Check sheet for the modelled part. Datum: model origin and axes. Units: mm. Round coordinates to 2 decimals unless told otherwise and drop trailing zeros. Loops run counter-clockwise (first coordinate to the right, second up) from the corner with the lowest first, then second, coordinate; pieces in that order, holes last. Notation, with made-up numbers: (6, -33.75) - (22, -33.75) arc R24 cw to (22, -17.75) - close; hole circle Ø5 at (-5, 16). An arc over 180 degrees is marked (long way). Put each result on its own line as item: value.
```python
from build123d import *

# Parameters (mm, degrees)
SKETCH1_W           = 115
SKETCH1_H           = 15
BOSS_EXTRUDE1_DEPTH = 0.5
SKETCH2_W           = 115
SKETCH2_H           = 10
CUT_EXTRUDE1_DEPTH  = 0.1
SKETCH3_W           = 0.4
SKETCH3_H           = 10
CUT_EXTRUDE2_DEPTH  = 0.4
LPATTERN3_COUNT     = 150
LPATTERN3_PITCH     = 0.8
SKETCH4_W           = 115
SKETCH4_H           = 5
BOSS_EXTRUDE2_DEPTH = 1
SKETCH5_W           = 77.289086501
SKETCH5_H           = 15.822063322
CUT_EXTRUDE3_DEPTH  = 1
SKETCH6_W           = 3.197112069
SKETCH6_H           = 15.066627115
CUT_EXTRUDE4_DEPTH  = 1
SKETCH7_W           = 3.877656405
SKETCH7_H           = 15.126214191
CUT_EXTRUDE7_DEPTH  = 1


with BuildPart() as part:
    # Sketch1 → Boss-Extrude1 (new body)
    with BuildSketch(Plane(origin=(0, 0, 0), x_dir=(1, 0, 0), z_dir=(0, 1, 0))):
        with Locations((57.5, 7.5)):
            Rectangle(SKETCH1_W, SKETCH1_H)
    extrude(amount=BOSS_EXTRUDE1_DEPTH)

    # Sketch2 → Cut-Extrude1 (cut)
    with BuildSketch(Plane(origin=(0, 0.5, 0), x_dir=(1, 0, 0), z_dir=(0, 1, 0))):
        with Locations((57.5, 10)):
            Rectangle(SKETCH2_W, SKETCH2_H)
    extrude(amount=-CUT_EXTRUDE1_DEPTH, mode=Mode.SUBTRACT)

    # Sketch3 → Cut-Extrude2 (cut)
    with BuildSketch(Plane(origin=(0, 0.4, 0), x_dir=(1, 0, 0), z_dir=(0, 1, 0))):
        with Locations((0.2, 10)):
            Rectangle(SKETCH3_W, SKETCH3_H)
    cut_extrude2 = extrude(amount=-CUT_EXTRUDE2_DEPTH, mode=Mode.SUBTRACT)

    # LPattern3: Cut-Extrude2 ×150
    with Locations(*[(i * LPATTERN3_PITCH, 0, 0) for i in range(1, LPATTERN3_COUNT)]):
        add(cut_extrude2, mode=Mode.SUBTRACT)

    # Sketch4 → Boss-Extrude2 (add)
    with BuildSketch(Plane.XZ):
        with Locations((57.5, -2.5)):
            Rectangle(SKETCH4_W, SKETCH4_H)
    extrude(amount=-BOSS_EXTRUDE2_DEPTH)

    # Sketch5 → Cut-Extrude3 (cut)
    with BuildSketch(Plane(origin=(0, 1, 0), x_dir=(1, 0, 0), z_dir=(0, 1, 0))):
        with Locations((38.64454325, 7.911031661)):
            Rectangle(SKETCH5_W, SKETCH5_H)
    extrude(amount=-CUT_EXTRUDE3_DEPTH, mode=Mode.SUBTRACT)

    # Sketch6 → Cut-Extrude4 (cut)
    with BuildSketch(Plane(origin=(0, 1, 0), x_dir=(1, 0, 0), z_dir=(0, 1, 0))):
        with Locations((78.887642535, 7.533313558)):
            Rectangle(SKETCH6_W, SKETCH6_H)
    extrude(amount=-CUT_EXTRUDE4_DEPTH, mode=Mode.SUBTRACT)

    # Sketch7 → Cut-Extrude7 (cut)
    with BuildSketch(Plane(origin=(0, 1, 0), x_dir=(1, 0, 0), z_dir=(0, 1, 0))):
        with Locations((82.425026773, 7.563107096)):
            Rectangle(SKETCH7_W, SKETCH7_H)
    extrude(amount=-CUT_EXTRUDE7_DEPTH, mode=Mode.SUBTRACT)


solid = part.part
```
Item 1: Go/stop test with a flat-tipped pin: pin 1 (3 mm diameter, centred on x = 95, z = -11, fed in from +Y). Record where the tip stops, or that it passes through.
Filled sheet:
pin 1: y = 0.4
Item 2: Section check B-B on y = 0.85. Enter the section's corners in (x, z), then the cut area to 3 significant figures.
Filled sheet:
outline: (84.36, -5) - (115, -5) - (115, 0) - (84.36, 0) - close
area: 153 mm²
Item 3: Release check for a two-part mould opening along X. For faces 1 (the flat face through (115, 0.2, -5.9)), 2 (the flat face through (99.5, 0.6, -5)), 3 (the flat face through (99, 1, -2)), 4 (the flat face through (84.364, 0.5, -2.5)) record: +X half, -X half, draft (parallel to the pull), parting line (faces both ways), or undercut.
Filled sheet:
face 1: +X half
face 2: undercut
face 3: draft
face 4: -X half
Item 4: Thickness scan on line 1 (Z direction, x = 96, y = 0.45); line 2 (Y direction, x = 92.5, z = -13.5). Record the ranges inside material, lowest first. Write a range as from..to.
Filled sheet:
line 1: -5..0
line 2: 0..0.4
Item 5: Section check A-A on z = -6. Count the separate pieces of the cut face and the enclosed holes in it, then the cut area to 3 significant figures.
Filled sheet:
separate pieces: 39
enclosed holes: 0
area: 6.16 mm²
